Source: CAD feature listing. Evaluate the final solid. Frame: model axes, mm. Face numbers are marked on the shaded views. A direction names the side the tool comes from. Round coordinates to 2 decimals unless told otherwise and drop trailing zeros. Write each loop counter-clockwise with the first axis right and the second up, starting at its lowest first coordinate (ties: lowest second). Pieces come first, ordered by that corner, then holes.
from build123d import *

# Parameters (mm, degrees)
SKETCH_W    = 104
SKETCH_H    = 34
PAD_DEPTH   = 40
THICKNESS_T = -2


with BuildPart() as part:
    # Sketch → Pad (new body)
    with BuildSketch(Plane.XY):
        Rectangle(SKETCH_W, SKETCH_H)
    extrude(amount=PAD_DEPTH)

    # Thickness
    thickness_openings = [part.faces().sort_by_distance(p)[0] for p in [
        (0, 0, 40),
    ]]
    offset(amount=THICKNESS_T, openings=thickness_openings)


solid = part.part
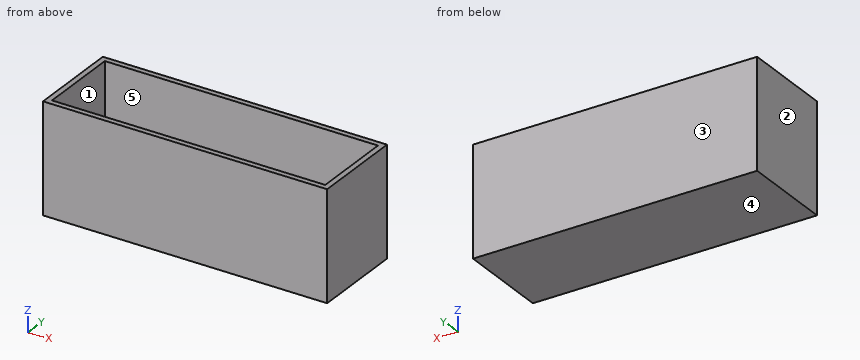
1) Contact query for flat-ended pins moving along their axis: P1, Ø2, axis at x = -41, y = -8, coming from the -Z side; P2, Ø1, axis at x = -40, y = -10, coming from the +Z side. Output: stop coordinate, or through.
Taken from the geometry:
P1: stops at z = 0
P2: stops at z = 2
2) Section query A-A on x = -25. Return the cut outline in (y, z).
Taken from the geometry:
outline: (-17, 0) - (17, 0) - (17, 40) - (15, 40) - (15, 2) - (-15, 2) - (-15, 40) - (-17, 40) - close
3) Section query C-C on y = 8. Return the cut outline in (x, z).
Taken from the geometry:
outline: (-52, 0) - (52, 0) - (52, 40) - (50, 40) - (50, 2) - (-50, 2) - (-50, 40) - (-52, 40) - close
4) Material intervals for line 1 (X direction, y = 7, z = 9); line 2 (Y direction, x = -14, z = 37); line 3 (Z direction, x = 31, y = 14), sorted ascending.
Taken from the geometry:
line 1: x = -52 to -50, 50 to 52
line 2: y = -17 to -15, 15 to 17
line 3: z = 0 to 2
5) Pull-direction query (Y, two-part tool) for the marked faces 3, 4 and 5; classes: released by +Y, released by -Y, zero draft, split by the parting line, or undercut.
Taken from the geometry:
face 3: released by +Y
face 4: zero draft
face 5: undercut
6) Reachability of the marked faces 1 and 2 from +Z, -Z, +X, -X, +Y, -Y: full face, straight path, thin tool, end or side. Return the list, or none.
Taken from the geometry:
face 1: +Z
face 2: +Z, -Z, -X, +Y, -Y
7) Section query B-B on z = 24.5. Return the cut outline in (x, y), then the cut area to 3 significant figures.
Taken from the geometry:
outline: (-52, -17) - (52, -17) - (52, 17) - (-52, 17) - close; hole (-50, -15) - (50, -15) - (50, 15) - (-50, 15) - close
area: 536 mm2
